from build123d import *

# Parameters (mm, degrees)
BOX001_W     = 10
BOX001_H     = 10
BOX001_DEPTH = 6
BOX002_W     = 10
BOX002_H     = 10
BOX002_DEPTH = 6
BOX003_W     = 110
BOX003_H     = 75
BOX003_DEPTH = 3
BOX004_W     = 10
BOX004_H     = 10
BOX004_DEPTH = 6
BOX005_W     = 10
BOX005_H     = 10
BOX005_DEPTH = 6
BOX_W        = 110
BOX_H        = 75
BOX_DEPTH    = 3


with BuildPart() as cube001:
    # Box001 → Box001 (new body)
    with BuildSketch(Plane.XY):
        with Locations((5, 5)):
            Rectangle(BOX001_W, BOX001_H)
    extrude(amount=BOX001_DEPTH)


with BuildPart() as cube002:
    # Box002 → Box002 (new body)
    with BuildSketch(Plane(origin=(0, 65, 0), x_dir=(1, 0, 0), z_dir=(0, 0, 1))):
        with Locations((5, 5)):
            Rectangle(BOX002_W, BOX002_H)
    extrude(amount=BOX002_DEPTH)


with BuildPart() as cube003:
    # Box003 → Box003 (new body)
    with BuildSketch(Plane.XY):
        with Locations((55, 37.5)):
            Rectangle(BOX003_W, BOX003_H)
    extrude(amount=BOX003_DEPTH)


with BuildPart() as cube004:
    # Box004 → Box004 (new body)
    with BuildSketch(Plane(origin=(100, 65, 0), x_dir=(1, 0, 0), z_dir=(0, 0, 1))):
        with Locations((5, 5)):
            Rectangle(BOX004_W, BOX004_H)
    extrude(amount=BOX004_DEPTH)


with BuildPart() as cube005:
    # Box005 → Box005 (new body)
    with BuildSketch(Plane(origin=(100, 0, 0), x_dir=(1, 0, 0), z_dir=(0, 0, 1))):
        with Locations((5, 5)):
            Rectangle(BOX005_W, BOX005_H)
    extrude(amount=BOX005_DEPTH)


with BuildPart() as fusion:
    # Box → Box (new body)
    with BuildSketch(Plane.XY):
        with Locations((55, 37.5)):
            Rectangle(BOX_W, BOX_H)
    extrude(amount=BOX_DEPTH)

    # Fusion: union Cube001, Cube002, Cube003, Cube004, Cube005
    add(cube001.part)
    add(cube002.part)
    add(cube003.part)
    add(cube004.part)
    add(cube005.part)


solid = fusion.part
Build history of the part. All positions in model axes, mm. A direction names the side the tool comes from. Round coordinates to 2 decimals unless told otherwise and drop trailing zeros. Write each loop counter-clockwise with the first axis right and the second up, starting at its lowest first coordinate (ties: lowest second). Pieces come first, ordered by that corner, then holes. Notation, with made-up numbers: (-0.5, 54) - (23.5, 54) arc R26 cw to (23.5, 93) - close; hole circle Ø8 at (76, 34.5). An arc over 180 degrees is marked (long way). One line per question, with ' | ' between items.
1. Band-saw the part on A-A, the plane z = 4.25. Write the cut outline in (x, y).
Results are:
outline: (0, 0) - (10, 0) - (10, 10) - (0, 10) - close; (0, 65) - (10, 65) - (10, 75) - (0, 75) - close; (100, 0) - (110, 0) - (110, 10) - (100, 10) - close; (100, 65) - (110, 65) - (110, 75) - (100, 75) - close
2. Tool access for faces 4 (the face through (105, 65, 4)), 5 (the face through (54, 0, 2)), 6 (the face through (100, 5, 4)): list every direction of +Z, -Z, +X, -X, +Y, -Y with a clear straight run to the whole face (end or side of a thin tool).
Results are:
face 4: +Z, +X, -X | face 5: +Z, -Z, +X, -X, -Y | face 6: +Z, +Y, -Y
3. Drop flat-ended pins along their axis: pin 1 Ø3.5 at (x, z) = (103, 4.5) entering from -Y; pin 2 Ø8 at (x, y) = (24, 24.5) entering from +Z. Give the stop position or say it passes through.
Results are:
pin 1: y = 0 | pin 2: z = 3
4. Band-saw the part on C-C, the plane x = 84. Write the cut outline in (y, z).
Results are:
outline: (0, 0) - (75, 0) - (75, 3) - (0, 3) - close
5. Drill centre lines: line 1 along Z through (x, y) = (81, 42); line 2 along Y through (x, z) = (6.5, 5.35). Where is each one in solid material? Low to high. Write a range as from..to.
Results are:
line 1: 0..3 | line 2: 0..10, 65..75
6. Mould opens along Y. For faces 1 (the face through (5, 5, 6)), 2 (the face through (105, 10, 4)), 3 (the face through (54, 75, 2)) say: released by +Y, released by -Y, zero draft, split by the parting line, or undercut.
Results are:
face 1: zero draft | face 2: undercut | face 3: released by +Y
7. Band-saw the part on B-B, the plane y = 25.5. Write the cut outline in (x, z).
Results are:
outline: (0, 0) - (110, 0) - (110, 3) - (0, 3) - close
